Here's the drawing with two shaded views (mm, measured from the low corner). I have some questions. Round coordinates to 2 decimals unless told otherwise and drop trailing zeros. Loops run counter-clockwise (first coordinate to the right, second up) from the corner with the lowest first, then second, coordinate; pieces in that order, holes last.
(1) I want a section at B-B on x = 28. Write out the boundary of the cut face in (y, z), plus the area to 3 significant figures.
(2) I want a section at A-A on y = 50. Write out the boundary of the cut face in (x, z), plus the area to 3 significant figures.
(3) Will this pin go through, and if not, where does the flat tip stop? pin 1 Ø12 at (x, z) = (21.5, 22) entering from +Y.
(4) I want a section at C-C on z = 31. Write out the boundary of the cut face in (x, y).
(5) If I drill on line 1 along Y through (x, z) = (27.5, 46.5); line 2 along Y through (x, z) = (42.5, 36); line 3 along Z through (x, y) = (20.5, 418.5), over which ranges is the centre line in solid material (lowest first)?
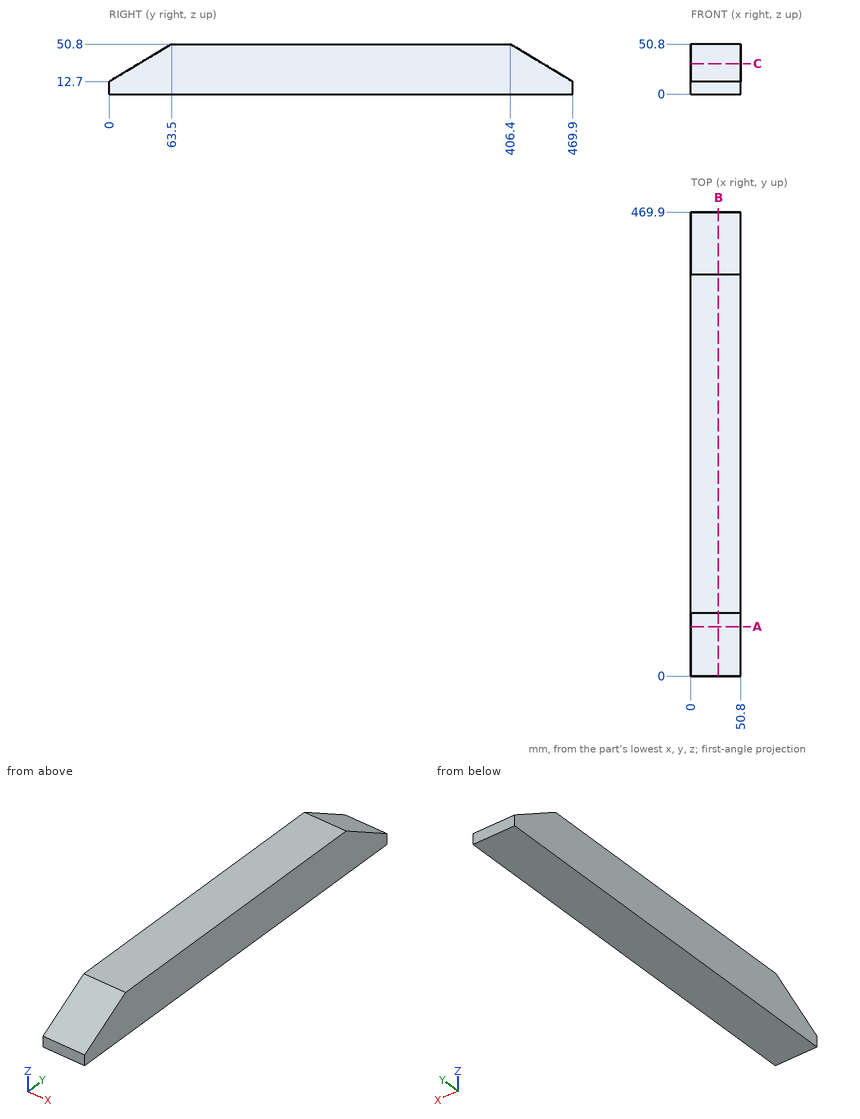
Filled sheet:
1. outline: (0, 0) - (469.9, 0) - (469.9, 12.7) - (406.4, 50.8) - (63.5, 50.8) - (0, 12.7) - close
1. area: 21,500 mm2
2. outline: (0, 0) - (50.8, 0) - (50.8, 42.7) - (0, 42.7) - close
2. area: 2,170 mm2
3. pin 1: stops at y = 464.4
4. outline: (0, 30.5) - (50.8, 30.5) - (50.8, 439.4) - (0, 439.4) - close
5. line 1: y = 56.33 to 413.57
5. line 2: y = 38.83 to 431.07
5. line 3: z = 0 to 43.54
